from build123d import *

# Parameters (mm, degrees)
SKETCH1_R              = 2.35
PIN_DEPTH              = 11.35
SKETCH2_R              = 2.95
MIDDLE_DEPTH           = 4.8
SKETCH3_R              = 2.625
OUTER_RIM_DEPTH        = 0.5
BORE_CUT_DEPTH         = 13.562941535
BORE_CUT_DEPTH_BACK    = 13.562941535
SLOT_CUT_DEPTH         = 13.562941535
SLOT_CUT_DEPTH_BACK    = 13.562941535
SKETCH6_R              = 3.7
MIDDLE_BODY_DEPTH      = 3.9
MIDDLE_BORE_DEPTH      = 14.012398084
MIDDLE_BORE_DEPTH_BACK = 14.012398084
SKETCH7_R              = 2.4
SKETCH8_R              = 3.05
MIDDLE_RIM_CUT_DEPTH   = 0.75


with BuildPart() as part:
    # Sketch1 → Pin (new, symmetric)
    with BuildSketch(Plane(origin=(0, 0, 0), x_dir=(0, 0, -1), z_dir=(1, 0, 0))):
        Circle(SKETCH1_R)
    extrude(amount=PIN_DEPTH, both=True)

    # Sketch2 → Middle (add, symmetric)
    with BuildSketch(Plane(origin=(0, 0, 0), x_dir=(0, 0, -1), z_dir=(1, 0, 0))):
        Circle(SKETCH2_R)
    extrude(amount=MIDDLE_DEPTH, both=True)

    # Sketch3 → Outer Rim (add)
    with BuildSketch(Plane(origin=(11.35, 0, 0), x_dir=(0, 0, -1), z_dir=(1, 0, 0))):
        Circle(SKETCH3_R)
    outer_rim = extrude(amount=OUTER_RIM_DEPTH)

    # Mirror1: Outer Rim across plane
    add(outer_rim.mirror(Plane(origin=(0, 0, 0), x_dir=(0, 0, 1), z_dir=(1, 0, 0))))

    # Sketch4 → Bore Cut (cut, two sides: drawn at the far end of the back side and taken through both)
    with BuildSketch(Plane(origin=(0, 0, 0), x_dir=(0, 0, -1), z_dir=(1, 0, 0)).offset(-BORE_CUT_DEPTH_BACK)):
        with BuildLine():
            ThreePointArc((-1.1, -1.393063172), (0, -1.775), (1.1, -1.393063172))
            Line((1.1, -1.393063172), (1.1, 1.393063172))
            ThreePointArc((1.1, 1.393063172), (0, 1.775), (-1.1, 1.393063172))
            Line((-1.1, 1.393063172), (-1.1, -1.393063172))
        make_face()
    extrude(amount=BORE_CUT_DEPTH + BORE_CUT_DEPTH_BACK, mode=Mode.SUBTRACT)

    # Sketch5 → Slot Cut (cut, two sides: drawn at the far end of the back side and taken through both)
    with BuildSketch(Plane.XY.offset(-SLOT_CUT_DEPTH_BACK)):
        with BuildLine():
            Line((14.3, -0.5), (9.4, -0.5))
            ThreePointArc((9.4, -0.5), (8.9, 0), (9.4, 0.5))
            Line((9.4, 0.5), (14.3, 0.5))
            ThreePointArc((14.3, 0.5), (14.8, 0), (14.3, -0.5))
        make_face()
        with BuildLine():
            Line((-14.3, -0.5), (-9.4, -0.5))
            ThreePointArc((-9.4, -0.5), (-8.9, 0), (-9.4, 0.5))
            Line((-9.4, 0.5), (-14.3, 0.5))
            ThreePointArc((-14.3, 0.5), (-14.8, 0), (-14.3, -0.5))
        make_face()
    extrude(amount=SLOT_CUT_DEPTH + SLOT_CUT_DEPTH_BACK, mode=Mode.SUBTRACT)

    # Sketch6 → Middle Body (add, symmetric)
    with BuildSketch(Plane.XY):
        Circle(SKETCH6_R)
    extrude(amount=MIDDLE_BODY_DEPTH, both=True)

    # Sketch7 → Middle Bore (cut, two sides: drawn at the far end of the back side and taken through both)
    with BuildSketch(Plane.XY.offset(-MIDDLE_BORE_DEPTH_BACK)):
        Circle(SKETCH7_R)
    extrude(amount=MIDDLE_BORE_DEPTH + MIDDLE_BORE_DEPTH_BACK, mode=Mode.SUBTRACT)

    # Sketch8 → Middle Rim Cut (cut)
    with BuildSketch(Plane.XY.offset(3.9)):
        Circle(SKETCH8_R)
    middle_rim_cut = extrude(amount=-MIDDLE_RIM_CUT_DEPTH, mode=Mode.SUBTRACT)

    # Mirror2: Middle Rim Cut across plane
    add(middle_rim_cut.mirror(Plane.XY), mode=Mode.SUBTRACT)


solid = part.part
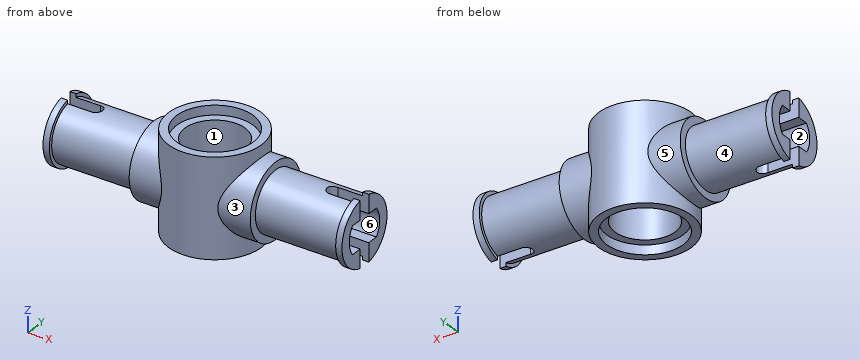
Model file for the job. Use its own axes, mm. Face numbers are marked on the shaded views. A direction names the side the tool comes from. Give positions to 0.01 mm unless a question says otherwise; leave off trailing zeros. Order: outer loops, then holes, each group sorted by start corner. A loop starts at its lowest first (then second) coordinate and runs counter-clockwise, first axis right, second up. Notation, with made-up numbers: M -36.75,75.5 L 19.25,75.5 A35 ccw 19.25,114.5 Z; hole C 27,58.5 d8. An arc over 180 degrees is marked long. Put each result on its own line as item: value. Start each with the question number.
(1) Drill centre lines: L1, parallel to X at y = 2.5, z = 0.5; L2, parallel to Y at x = 0, z = 3.75; L3, parallel to Y at x = 0, z = 1.75. Where is each one in solid material? Low to high. Write a range as [from, to].
(2) Pin check, flat tips, straight feed: pin 1 Ø1.5 at (x, z) = (8.5, 1.5) entering from -Y; pin 2 Ø0.7 at (x, z) = (10.5, 2) entering from -Y; pin 3 Ø1.6 at (x, z) = (-11, -2) entering from +Y. Stop position of each tip, or through.
(3) Pull direction Y, two halves, no side cores. Call the marked faces 1, 2 and 3: released by +Y, released by -Y, zero draft, split by the parting line, or undercut.
(4) Band-saw the part on C-C on x = -8.5. Give the cut face in (y, z) (3 decimals), then the cut area to 3 significant figures.
(5) Tool access for the marked faces 4, 5 and 6: list every direction of +Z, -Z, +X, -X, +Y, -Y with a clear straight run to the whole face (end or side of a thin tool).
(6) Band-saw the part on A-A on x = 0. Give the cut face in (y, z), then the cut area to 3 significant figures.
Results below:
1. L1: x = [-11.85, -11.35], [-4.8, 4.8], [11.35, 11.85]
1. L2: y = [-3.7, -3.05], [3.05, 3.7]
1. L3: y = [-3.7, -2.4], [2.4, 3.7]
2. pin 1: stops at y = -2.23
2. pin 2: stops at y = -1.67
2. pin 3: stops at y = 2.29
3. face 1: undercut
3. face 2: undercut
3. face 3: split by the parting line
4. outline: C 0,0 d4.7; hole M -1.393,-1.1 L 1.393,-1.1 A1.775 ccw 1.393,1.1 L -1.393,1.1 A1.775 ccw Z
4. area: 10.1 mm2
5. face 4: none
5. face 5: -X
5. face 6: +X
6. outline: M -3.7,-3.9 L -3.05,-3.9 L -3.05,-3.15 L -2.4,-3.15 L -2.4,3.15 L -3.05,3.15 L -3.05,3.9 L -3.7,3.9 Z; M 2.4,-3.15 L 3.05,-3.15 L 3.05,-3.9 L 3.7,-3.9 L 3.7,3.9 L 3.05,3.9 L 3.05,3.15 L 2.4,3.15 Z
6. area: 18.3 mm2
